```python
from build123d import *

# Parameters (mm, degrees)
EXTRUDE2_DEPTH      = 10
EXTRUDE3_DEPTH      = 5
CUT_EXTRUDE1_DEPTH  = 5
EXTRUDE4_DEPTH      = 3
CUT_EXTRUDE2_DEPTH  = 8
EXTRUDE5_DEPTH      = 5
EXTRUDE5_DEPTH_BACK = 5
CUT_EXTRUDE3_DEPTH  = 5
SKETCH9_W           = 5
SKETCH9_H           = 15
EXTRUDE6_DEPTH      = 35
SKETCH11_W          = 5
SKETCH11_H          = 35
EXTRUDE8_DEPTH      = 25
EXTRUDE9_DEPTH      = 25
EXTRUDE12_DEPTH     = 20
EXTRUDE13_DEPTH     = 5
CUT_EXTRUDE5_DEPTH  = 5
EXTRUDE14_DEPTH     = 10
EXTRUDE19_DEPTH     = 5
SKETCH21_R          = 0.7
EXTRUDE20_DEPTH     = 0.5


with BuildPart() as part:
    # Sketch2 → Extrude2 (new body)
    with BuildSketch(Plane.XY):
        with BuildLine():
            Line((-26.9875, 0), (-26.9875, -10))
            Line((-26.9875, -10), (-21.9875, -10))
            Line((-21.9875, -10), (-21.9875, 0))
            ThreePointArc((-21.9875, 0), (-15.547510351, 15.547510351), (0, 21.9875))
            ThreePointArc((0, 21.9875), (20.037638412, 13.687638412), (28.3375, -6.35))
            ThreePointArc((28.3375, -6.35), (16.317894533, -35.367894533), (-12.7, -47.3875))
            ThreePointArc((-12.7, -47.3875), (-55.188278715, -29.788278715), (-72.7875, 12.7))
            ThreePointArc((-72.7875, 12.7), (-47.748790957, 73.148790957), (12.7, 98.1875))
            ThreePointArc((12.7, 98.1875), (95.599431259, 63.849431259), (129.9375, -19.05))
            Line((129.9375, -19.05), (134.9375, -19.05))
            ThreePointArc((134.9375, -19.05), (99.134965165, 67.384965165), (12.7, 103.1875))
            ThreePointArc((12.7, 103.1875), (-51.284324863, 76.684324863), (-77.7875, 12.7))
            ThreePointArc((-77.7875, 12.7), (-58.72381262, -33.32381262), (-12.7, -52.3875))
            ThreePointArc((-12.7, -52.3875), (19.853428439, -38.903428439), (33.3375, -6.35))
            ThreePointArc((33.3375, -6.35), (23.573172318, 17.223172318), (0, 26.9875))
            ThreePointArc((0, 26.9875), (-19.083044257, 19.083044257), (-26.9875, 0))
        make_face()
    extrude(amount=EXTRUDE2_DEPTH)

    # Sketch3 → Extrude3 (add)
    with BuildSketch(Plane.XY):
        with BuildLine():
            Line((-21.9875, 0), (-21.9875, -10))
            Line((-21.9875, -10), (-31.9875, -10))
            Line((-31.9875, -10), (-31.9875, 0))
            ThreePointArc((-31.9875, 0), (-22.618578163, 22.618578163), (0, 31.9875))
            ThreePointArc((0, 31.9875), (27.108706224, 20.758706224), (38.3375, -6.35))
            ThreePointArc((38.3375, -6.35), (23.388962345, -42.438962345), (-12.7, -57.3875))
            ThreePointArc((-12.7, -57.3875), (-62.259346526, -36.859346526), (-82.7875, 12.7))
            ThreePointArc((-82.7875, 12.7), (-54.819858769, 80.219858769), (12.7, 108.1875))
            ThreePointArc((12.7, 108.1875), (102.670499071, 70.920499071), (139.9375, -19.05))
            Line((139.9375, -19.05), (129.9375, -19.05))
            ThreePointArc((129.9375, -19.05), (95.599431259, 63.849431259), (12.7, 98.1875))
            ThreePointArc((12.7, 98.1875), (-47.748790957, 73.148790957), (-72.7875, 12.7))
            ThreePointArc((-72.7875, 12.7), (-55.188278715, -29.788278715), (-12.7, -47.3875))
            ThreePointArc((-12.7, -47.3875), (16.317894533, -35.367894533), (28.3375, -6.35))
            ThreePointArc((28.3375, -6.35), (20.037638412, 13.687638412), (0, 21.9875))
            ThreePointArc((0, 21.9875), (-15.547510351, 15.547510351), (-21.9875, 0))
        make_face()
    extrude(amount=-EXTRUDE3_DEPTH)

    # Sketch4 → Cut-Extrude1 (cut)
    with BuildSketch(Plane.ZY.offset(26.9875)):
        Polygon((0, -10), (5, 0), (10, 0), (10, -10), align=None)
    extrude(amount=-CUT_EXTRUDE1_DEPTH, mode=Mode.SUBTRACT)

    # Sketch5 → Extrude4 (add)
    with BuildSketch(Plane(origin=(-21.9875, 0, 0), x_dir=(0, 0, -1), z_dir=(1, 0, 0))):
        Polygon((0, -10), (-5, 0), (0, 0), (5, 0), (5, -10), align=None)
    extrude(amount=EXTRUDE4_DEPTH)

    # Sketch6 → Cut-Extrude2 (cut)
    with BuildSketch(Plane(origin=(-18.9875, 0, 0), x_dir=(0, 0, -1), z_dir=(1, 0, 0))):
        Polygon((5, -5.5), (-2.25, -5.5), (0, -10), (5, -10), align=None)
    extrude(amount=-CUT_EXTRUDE2_DEPTH, mode=Mode.SUBTRACT)

    # Sketch7 → Extrude5 (add, two sides)
    with BuildSketch(Plane.ZY.offset(26.9875)) as extrude5_sk:
        Polygon((0, -5.5), (0.798113635, -5.5), (0, 14), align=None)
    extrude(amount=EXTRUDE5_DEPTH)
    extrude(extrude5_sk.sketch, amount=-EXTRUDE5_DEPTH_BACK)

    # Sketch8 → Cut-Extrude3 (cut)
    with BuildSketch(Plane.XY):
        with BuildLine():
            Line((-28.761087536, 14), (-31.9875, 14))
            Line((-31.9875, 14), (-31.9875, 0))
            ThreePointArc((-31.9875, 0), (-31.170462331, 7.183483441), (-28.761087536, 14))
        make_face()
    extrude(amount=CUT_EXTRUDE3_DEPTH, mode=Mode.SUBTRACT)

    # Sketch9 → Extrude6 (add)
    with BuildSketch(Plane.XZ.offset(19.05)):
        with Locations((132.4375, 2.5)):
            Rectangle(SKETCH9_W, SKETCH9_H)
    extrude(amount=EXTRUDE6_DEPTH)

    # Sketch11 → Extrude8 (add)
    with BuildSketch(Plane(origin=(0, 0, -5), x_dir=(-1, 0, 0), z_dir=(0, 0, -1))):
        with Locations((-132.4375, -36.55)):
            Rectangle(SKETCH11_W, SKETCH11_H)
    extrude(amount=EXTRUDE8_DEPTH)

    # Sketch12 → Extrude9 (add)
    with BuildSketch(Plane(origin=(0, 0, -5), x_dir=(-1, 0, 0), z_dir=(0, 0, -1))):
        with BuildLine():
            Line((-129.9375, -19.05), (-139.9375, -19.05))
            ThreePointArc((-139.9375, -19.05), (-139.918121112, -16.829399436), (-139.859990353, -14.609475288))
            Line((-139.859990353, -14.609475288), (-129.866082083, -14.958470255))
            ThreePointArc((-129.866082083, -14.958470255), (-129.919644161, -17.0039235), (-129.9375, -19.05))
        make_face()
    extrude(amount=EXTRUDE9_DEPTH)

    # Sketch16 → Extrude12 (add)
    with BuildSketch(Plane.XY.offset(10)):
        Polygon((129.9375, -19.05), (129.9375, -54.05), (139.9375, -54.05), (139.9375, -49.05), (134.9375, -49.05), (134.9375, -19.05), align=None)
    extrude(amount=EXTRUDE12_DEPTH)

    # Sketch17 → Extrude13 (add)
    with BuildSketch(Plane(origin=(134.9375, 0, 0), x_dir=(0, 0, -1), z_dir=(1, 0, 0))):
        Polygon((-10, -54.05), (-10, -49.05), (-5, -49.05), (30, -29.72873513), (30, -34.988734421), (-5, -54.05), align=None)
    extrude(amount=EXTRUDE13_DEPTH)

    # Sketch18 → Cut-Extrude5 (cut)
    with BuildSketch(Plane(origin=(134.9375, 0, 0), x_dir=(0, 0, -1), z_dir=(1, 0, 0))):
        Polygon((-5, -54.05), (30, -34.988734421), (30, -54.05), align=None)
        Polygon((-30, -19.05), (-30, -34.05), (-10, -22.05), (-10, -19.05), align=None)
    extrude(amount=-CUT_EXTRUDE5_DEPTH, mode=Mode.SUBTRACT)

    # Sketch19 → Extrude14 (add)
    with BuildSketch(Plane(origin=(0, 0, -30), x_dir=(-1, 0, 0), z_dir=(0, 0, -1))):
        Polygon((-134.9375, -19.05), (-134.9375, -29.72873513), (-120.74, -65.09), (-115.74, -65.09), (-129.9375, -29.72873513), (-129.866082083, -14.958470255), (-139.859990353, -14.609475288), (-139.9375, -19.05), align=None)
    extrude(amount=EXTRUDE14_DEPTH)

    # Sketch20 → Extrude19 (add)
    with BuildSketch(Plane.XY):
        with BuildLine():
            Line((128.760903372, -2.482015371), (38.141874641, -2.482015371))
            ThreePointArc((38.141874641, -2.482015371), (37.760120708, 0.278513435), (37.178841709, 3.004017073))
            Line((37.178841709, 3.004017073), (127.844482009, 3.004017073))
            ThreePointArc((127.844482009, 3.004017073), (128.335231203, 0.266436289), (128.760903372, -2.482015371))
        make_face()
        with BuildLine():
            Line((0, 31.9875), (0, 97.238882511))
            ThreePointArc((0, 97.238882511), (-3.385770157, 96.660470787), (-6.745571925, 95.946515776))
            Line((-6.745571925, 95.946515776), (-6.745571925, 31.268153378))
            ThreePointArc((-6.745571925, 31.268153378), (-3.391909497, 31.807154953), (0, 31.9875))
        make_face()
        with BuildLine():
            Line((-0.000749496, 21.987499987), (-0.000749496, 3.004017073))
            Line((-0.000749496, 3.004017073), (26.74913589, 3.004017073))
            ThreePointArc((26.74913589, 3.004017073), (27.547611511, 0.294020339), (28.072274599, -2.482015371))
            Line((28.072274599, -2.482015371), (0.080484541, -2.482015371))
            Line((0.080484541, -2.482015371), (0.080484541, -45.312306862))
            ThreePointArc((0.080484541, -45.312306862), (-3.298138872, -46.262230565), (-6.745571925, -46.919996909))
            Line((-6.745571925, -46.919996909), (-6.745571925, -2.482015371))
            Line((-6.745571925, -2.482015371), (-18.9875, -2.482015371))
            Line((-18.9875, -2.482015371), (-18.9875, 0))
            Line((-18.9875, 0), (-21.9875, 0))
            ThreePointArc((-21.9875, 0), (-21.928738235, 1.606423254), (-21.752767023, 3.20426015))
            Line((-21.752767023, 3.20426015), (-6.745571925, 3.004017073))
            Line((-6.745571925, 3.004017073), (-6.745571925, 20.92719321))
            ThreePointArc((-6.745571925, 20.92719321), (-3.414568171, 21.720747696), (-0.000749496, 21.987499987))
        make_face()
        with BuildLine():
            Line((-31.826606372, 3.20426015), (-50.922171332, 3.20426015))
            Line((-50.922171332, 3.20426015), (-72.032441219, 3.20426015))
            ThreePointArc((-72.032441219, 3.20426015), (-71.503716958, 0.345627166), (-70.83734731, -2.484087197))
            Line((-70.83734731, -2.484087197), (-50.922171332, -2.484087197))
            Line((-50.922171332, -2.484087197), (-31.9875, -2.484087197))
            Line((-31.9875, -2.484087197), (-31.9875, 0))
            ThreePointArc((-31.9875, 0), (-31.947251271, 1.604148518), (-31.826606372, 3.20426015))
        make_face()
        with BuildLine():
            Line((26.74913589, 21.11356924), (73.944333787, 80.918810062))
            ThreePointArc((73.944333787, 80.918810062), (71.049492521, 82.635633837), (68.106562726, 84.268653752))
            Line((68.106562726, 84.268653752), (21.610975976, 25.315906329))
            ThreePointArc((21.610975976, 25.315906329), (24.271176613, 23.326150223), (26.74913589, 21.11356924))
        make_face()
    extrude(amount=-EXTRUDE19_DEPTH)

    # Sketch21 → Extrude20 (add)
    with BuildSketch(Plane(origin=(0, -2, 4), x_dir=(1, 0, 0), z_dir=(0, -0.447213595, 0.894427191))):
        with Locations((-23.8075, -1)):
            Circle(SKETCH21_R)
        with Locations((-20.6275, -1)):
            Circle(SKETCH21_R)
    extrude(amount=EXTRUDE20_DEPTH)


solid = part.part
```
Can you work these out from the model? Positions are in its coordinate system, mm. A direction names the side the tool comes from. Coordinates: 2 decimals unless noted, no trailing zeros. Loops run counter-clockwise (first coordinate to the right, second up) from the corner with the lowest first, then second, coordinate; pieces in that order, holes last.
Item 1: I'm going to push flat-ended pins straight in: pin 1 (10 mm diameter, centred on y = 87.5, z = 18.5, fed in from +X); pin 2 (5.5 mm diameter, centred on y = 70.5, z = -1.5, fed in from -X); pin 3 (8 mm diameter, centred on x = 137.5, z = 19, fed in from -Y); pin 4 (3 mm diameter, centred on x = 65, y = 69.5, fed in from -Z). Where does each tip first touch, or does it pass through?
Answers below:
pin 1: passes through
pin 2: stops at x = -65.32
pin 3: stops at y = -54.05
pin 4: stops at z = -5
Item 2: If we mould it in two halves opening along X, with no side actions, what happens to faces 1 (the face through (134.87, -44.39, -12.74)), 2 (the face through (13, 3.004, -2)), 3 (the face through (134.938, -34, -5))? For each: released by +X, released by -X, zero draft, split by the parting line, or undercut.
Answers below:
face 1: zero draft
face 2: undercut
face 3: released by +X
Item 3: Suppose I cut it at A-A (x = 99.5). Please give me the cut outline in (y, z), then the cut area to 3 significant figures.
Answers below:
outline: (-2.48, -5) - (3, -5) - (3, 0) - (-2.48, 0) - close; (59.76, -5) - (73.98, -5) - (73.98, 0) - (67.02, 0) - (67.02, 10) - (59.76, 10) - close
area: 171 mm2
Item 4: Suppose I cut it at C-C (z = 22.5). Please give me the cut outline in (x, y), then the cut area to 4 significant figures.
Answers below:
outline: (129.94, -54.05) - (139.94, -54.05) - (139.94, -49.05) - (134.94, -49.05) - (134.94, -29.55) - (129.94, -29.55) - close
area: 147.5 mm2
Item 5: Suppose I cut it at B-B (y = 40). Please give me the cut outline in (x, z).
Answers below:
outline: (-78.8, -5) - (-68.31, -5) - (-68.31, 10) - (-73.57, 10) - (-73.57, 0) - (-78.8, 0) - close; (-6.75, -5) - (0, -5) - (0, 0) - (-6.75, 0) - close; (33.19, -5) - (41.65, -5) - (41.65, 0) - (33.19, 0) - close; (113.98, -5) - (125.41, -5) - (125.41, 0) - (119.73, 0) - (119.73, 10) - (113.98, 10) - close
Item 6: Which directions (+Z, -Z, +X, -X, +Y, -Y) give clear straight access to the entire face, cutting with the end or side of a thin tool? Please do faces 4 (the face through (-6.746, 64, -2)), 5 (the face through (19.494, -39.259, 4.93)), 6 (the face through (20, 26, 0)), 7 (the face through (137, -19.05, -20)).
Answers below:
face 4: +Z, -Z
face 5: +Z, -Y
face 6: +Z
face 7: +Z, -Z, +X
Item 7: Please list where these lines run through material, in increasing order: L1, parallel to X at y = 35, z = -0.5; L2, parallel to X at y = -18.5, z = -9; L3, parallel to Z at x = -8.5, y = 26.
Answers below:
L1: x = -80.15 to -69.83, -6.75 to 0, 29.25 to 37.71, 116.73 to 127.89
L2: x = 129.94 to 139.94
L3: z = -5 to 0
Item 8: Suppose I cut it at D-D (x = -46.5). Please give me the cut outline in (y, z).
Answers below:
outline: (-48.7, -5) - (-36.98, -5) - (-36.98, 10) - (-42.92, 10) - (-42.92, 0) - (-48.7, 0) - close; (-2.48, -5) - (3.2, -5) - (3.2, 0) - (-2.48, 0) - close; (74.37, -5) - (87.62, -5) - (87.62, 0) - (81.13, 0) - (81.13, 10) - (74.37, 10) - close
